Work out the finished part from the listing and answer in its coordinate system (mm). Face numbers are marked on the shaded views. A direction names the side the tool comes from. Round coordinates to 2 decimals unless told otherwise and drop trailing zeros. Order: outer loops, then holes, each group sorted by start corner. A loop starts at its lowest first (then second) coordinate and runs counter-clockwise, first axis right, second up. Notation, with made-up numbers: M 65.25,58 L 81.25,58 A28 cw 81.25,80 Z; hole C 8,51.5 d8. An arc over 180 degrees is marked long. Return JSON: item names as keys, results as strings.
from build123d import *

# Parameters (mm, degrees)
F1_DEPTH = 120
F4_W     = 10
F4_H     = 10
F5_DEPTH = 150
F6_D     = 9
F6_DEPTH = 15
F6_TIP   = 2.7038727856
F7_R     = 5


# Not quite as in the source:
# - a feature names something its author has since deleted; it is built from what else it names


with BuildPart() as f1:
    # F0 (on Top) → F1 (new body)
    with BuildSketch(Plane.XY):
        Polygon((100, -80), (100, 80), (-100, 80), (-100, -80), (-55, -80), (-30, -80), (-30, -10), (-30, 20), (30, 20), (30, -16.3740634173), (30, -80), (55, -80), align=None)
    extrude(amount=F1_DEPTH)

    # F4 (on face) → F5 (join)
    with BuildSketch(Plane(origin=(0, 80, 0), x_dir=(-1, 0, 0), z_dir=(0, 1, 0))):
        with Locations((95, 125)):
            Rectangle(F4_W, F4_H)
        with Locations((-95, 125)):
            Rectangle(F4_W, F4_H)
    extrude(amount=-F5_DEPTH)

    # F6
    with Locations(Plane(origin=(0, 0, 0), x_dir=(1, 0, 0), z_dir=(0, 0, -1))):
        with Locations((-80, -60), (-80, 60), (80, 60), (80, -60)):
            Hole(F6_D / 2, depth=F6_DEPTH)
            with Locations((0, 0, -(F6_DEPTH + F6_TIP / 2))):  # 118° drill point
                Cone(0, F6_D / 2, F6_TIP, mode=Mode.SUBTRACT)

    # F7
    f7_edges = [f1.edges().sort_by_distance(p)[0] for p in [
        (-30, 20, 60),
        (30, 20, 60),
    ]]
    fillet(f7_edges, radius=F7_R)


solid = f1.part
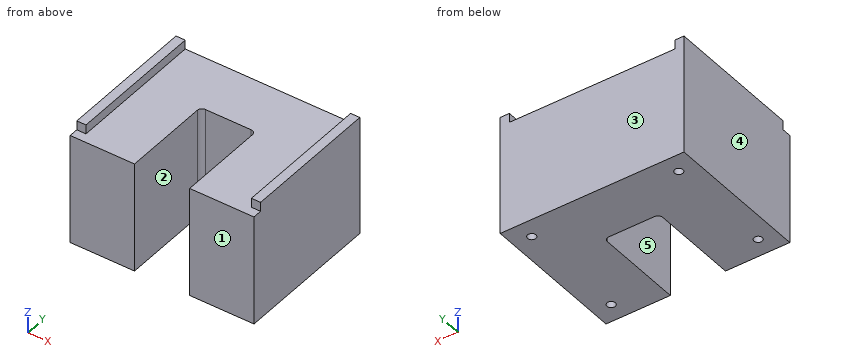
Item 1: Find section C-C (z = 114.5). Determine the outline of the cut face in (x, y), plus the area to 3 significant figures.
Output:
{"outline": "M -100,-80 L -30,-80 L -30,15 A5 cw -25,20 L 25,20 A5 cw 30,15 L 30,-80 L 100,-80 L 100,80 L -100,80 Z", "area": "26,000 mm^2"}
Item 2: Consider line 1 along Y through (x, z) = (80, 5.5); line 2 along X through (y, z) = (60, 5.75); line 3 along X through (y, z) = (-60, 7.5). Determine where each line is inside the solid, lowest interval first. Write a range as [from, to].
Output:
{"line 1": "y = [-80, -64.5], [-55.5, 55.5], [64.5, 80]", "line 2": "x = [-100, -84.5], [-75.5, 75.5], [84.5, 100]", "line 3": "x = [-100, -84.5], [-75.5, -30], [30, 75.5], [84.5, 100]"}
Item 3: Find section A-A (y = -4.5). Determine the outline of the cut face in (x, z).
Output:
{"outline": "M -100,0 L -30,0 L -30,120 L -90,120 L -90,130 L -100,130 Z; M 30,0 L 100,0 L 100,130 L 90,130 L 90,120 L 30,120 Z"}
Item 4: Which of the six approach directions +Z, -Z, +X, -X, +Y, -Y give full straight-line access (tool end or side, diameter ignored) to the marked faces 1 and 2?
Output:
{"face 1": "+Z, -Z, +X, -X, -Y", "face 2": "+Z, -Z, -Y"}
Item 5: The mould has two halves that part along X. Classify the marked faces 3, 4 and 5: pulls with the +X half, pulls with the -X half, needs draft (parallel to the pull), parting line crosses it, or undercut.
Output:
{"face 3": "needs draft", "face 4": "pulls with the -X half", "face 5": "undercut"}
Item 6: Each of these flat-tipped pins is pushed along its axis until it touches: pin 1 (5 mm diameter, centred on x = 13, y = 35, fed in from +Z); pin 2 (2 mm diameter, centred on x = -20, z = 80, fed in from -Y); pin 3 (5 mm diameter, centred on x = 93.5, z = 125, fed in from -Y). Where does it stop, or does it pass through?
Output:
{"pin 1": "stops at z = 120", "pin 2": "stops at y = 20", "pin 3": "stops at y = -70"}
Item 7: Find section B-B (y = 27). Determine the outline of the cut face in (x, z).
Output:
{"outline": "M -100,0 L 100,0 L 100,130 L 90,130 L 90,120 L -90,120 L -90,130 L -100,130 Z"}
Item 8: Find section D-D (x = 16). Determine the outline of the cut face in (y, z), plus the area to 3 significant figures.
Output:
{"outline": "M 20,0 L 80,0 L 80,120 L 20,120 Z", "area": "7,200 mm^2"}
